```python
from build123d import *

# Parameters (mm, degrees)
BASE_EXTRUDE_DEPTH  = 2.54
SKETCH2_W           = 9.525
SKETCH2_H           = 6.35
CUT_EXTRUDE1_DEPTH  = 0.508
SKETCH3_W           = 4.572
SKETCH3_H           = 6.35
BOSS_EXTRUDE1_DEPTH = 8.382
SKETCH4_R           = 1.5875
CUT_EXTRUDE2_DEPTH  = 19.230583479
SKETCH5_W           = 4.1402
SKETCH5_H           = 5.08
BOSS_EXTRUDE2_DEPTH = 4.826
BOSS_EXTRUDE3_DEPTH = 0.635
SKETCH7_R           = 0.127
BOSS_EXTRUDE4_DEPTH = 9.525


with BuildPart() as part:
    # Sketch1 → Base-Extrude (new body)
    with BuildSketch(Plane(origin=(0, 0, 0), x_dir=(1, 0, 0), z_dir=(0, 1, 0))):
        with BuildLine():
            Line((12.7, 3.175), (-12.7, 3.175))
            ThreePointArc((-12.7, 3.175), (-15.875, 0), (-12.7, -3.175))
            Line((-12.7, -3.175), (12.7, -3.175))
            ThreePointArc((12.7, -3.175), (15.875, 0), (12.7, 3.175))
        make_face()
    extrude(amount=BASE_EXTRUDE_DEPTH)

    # Sketch2 → Cut-Extrude1 (cut)
    with BuildSketch(Plane(origin=(0, 2.54, 0), x_dir=(-1, 0, 0), z_dir=(0, 1, 0))):
        Rectangle(SKETCH2_W, SKETCH2_H)
    extrude(amount=-CUT_EXTRUDE1_DEPTH, mode=Mode.SUBTRACT)

    # Sketch3 → Boss-Extrude1 (add)
    with BuildSketch(Plane(origin=(0, 2.54, 0), x_dir=(-1, 0, 0), z_dir=(0, 1, 0))):
        with Locations((-7.0485, 0)):
            Rectangle(SKETCH3_W, SKETCH3_H)
        with Locations((7.0485, 0)):
            Rectangle(SKETCH3_W, SKETCH3_H)
    extrude(amount=BOSS_EXTRUDE1_DEPTH)

    # Sketch4 → Cut-Extrude2 (cut, through all)
    with BuildSketch(Plane(origin=(0, 2.54, 0), x_dir=(-1, 0, 0), z_dir=(0, 1, 0))):
        with Locations(Location((-12.7, 0, 0), (0, 0, 90))):
            Circle(SKETCH4_R)
        with Locations(Location((12.7, 0, 0), (0, 0, 270))):
            Circle(SKETCH4_R)
    extrude(amount=-CUT_EXTRUDE2_DEPTH, mode=Mode.SUBTRACT)

    # Sketch5 → Boss-Extrude2 (add)
    with BuildSketch(Plane.XZ):
        with Locations((6.1341, 0)):
            Rectangle(SKETCH5_W, SKETCH5_H)
        with Locations((-6.1341, 0)):
            Rectangle(SKETCH5_W, SKETCH5_H)
    extrude(amount=BOSS_EXTRUDE2_DEPTH)

    # Sketch6 → Boss-Extrude3 (add, symmetric)
    with BuildSketch(Plane.XY):
        with BuildLine():
            Line((-4.064, 0), (4.064, 0))
            Line((4.064, 0), (4.064, -3.305361967))
            ThreePointArc((4.064, -3.305361967), (0, -1.082087461), (-4.064, -3.305361967))
            Line((-4.064, -3.305361967), (-4.064, 0))
        make_face()
    extrude(amount=BOSS_EXTRUDE3_DEPTH, both=True)

    # Sketch7 → Boss-Extrude4 (add)
    with BuildSketch(Plane.ZY.offset(-4.7625)):
        with Locations(Location((0, 8.128, 0), (0, 0, 180))):
            Circle(SKETCH7_R)
    extrude(amount=BOSS_EXTRUDE4_DEPTH)


solid = part.part
```
Geometry: final body of the model. Coordinates: model frame, mm. A direction names the side the tool comes from. Round coordinates to 2 decimals unless told otherwise and drop trailing zeros. Write each loop counter-clockwise with the first axis right and the second up, starting at its lowest first coordinate (ties: lowest second). Pieces come first, ordered by that corner, then holes.
Item 1: Pin query (flat end, axial travel): P1, Ø1.2, axis at x = -6.5, y = -3, coming from the -Z side; P2, Ø2.5, axis at y = -2, z = -1, coming from the -X side; P3, Ø1, axis at x = 10.5, z = -0.5, coming from the -Y side. Return the tip coordinate at first contact, or that it passes through.
Item 2: Mould query, pull axis X, two halves, no side actions, for faces 1 (the face through (4.064, -3.5, 0)), 2 (the face through (-7, 10.922, 0)), 3 (the face through (-9.334, 7, 0)). Classes: +X half, -X half, draft (parallel to the pull), parting line (faces both ways), or undercut.
Item 3: Set-up query: faces 4 (the face through (6, -2, -2.54)), 5 (the face through (6, -2, 2.54)), 6 (the face through (-11, 2.54, 1)), 7 (the face through (9.334, 7, 0)), 8 (the face through (0.1, -0.9, 0.635)). Return all of +Z, -Z, +X, -X, +Y, -Y with unobstructed straight access to the full face (end or side cutting, diameter ignored); none if empty.
Item 4: Material intervals for L1, parallel to X at y = 1.45, z = 0 (1 decimal); L2, parallel to Z at x = -12.7, y = 1.1 (1 decimal); L3, parallel to X at y = -3.25, z = 2, sorted ascending.
Item 5: Section query B-B (z = -1). Return loops of the section in (x, y), plus the area to 3 significant figures.
Item 6: Section query D-D (y = -3). Return loops of the section in (x, z) (3 decimals).
Item 7: Section query C-C (x = -1). Return loops of the section in (y, z) (3 decimals).
Item 8: Section query A-A (y = 9.5). Return loops of the section in (x, z) (1 decimal), plus the area to 3 significant figures.
Completed:
1. P1: stops at z = -2.54
1. P2: stops at x = -8.2
1. P3: stops at y = 0
2. face 1: undercut
2. face 2: draft
2. face 3: -X half
3. face 4: -Z, +X, -X, -Y
3. face 5: +Z, +X, -X, -Y
3. face 6: +Z, -Z, -X, +Y
3. face 7: +Z, -Z, +X, +Y
3. face 8: +Z, -Y
4. L1: x = -15.9 to -14.3, -11.1 to 11.1, 14.3 to 15.9
4. L2: z = -3.2 to -1.6, 1.6 to 3.2
4. L3: x = -8.2 to -4.06, 4.06 to 8.2
5. outline: (-15.71, 0) - (-13.93, 0) - (-13.93, 2.54) - (-15.71, 2.54) - close; (-11.47, 0) - (-8.2, 0) - (-8.2, -4.83) - (-4.06, -4.83) - (-4.06, 0) - (4.06, 0) - (4.06, -4.83) - (8.2, -4.83) - (8.2, 0) - (11.47, 0) - (11.47, 2.54) - (9.33, 2.54) - (9.33, 10.92) - (4.76, 10.92) - (4.76, 2.03) - (-4.76, 2.03) - (-4.76, 10.92) - (-9.33, 10.92) - (-9.33, 2.54) - (-11.47, 2.54) - close; (13.93, 0) - (15.71, 0) - (15.71, 2.54) - (13.93, 2.54) - close
5. area: 179 mm2
6. outline: (-8.204, -2.54) - (-4.064, -2.54) - (-4.064, -0.635) - (-3.851, -0.635) - (-3.851, 0.635) - (-4.064, 0.635) - (-4.064, 2.54) - (-8.204, 2.54) - close; (3.851, -0.635) - (4.064, -0.635) - (4.064, -2.54) - (8.204, -2.54) - (8.204, 2.54) - (4.064, 2.54) - (4.064, 0.635) - (3.851, 0.635) - close
7. outline: (-1.187, -0.635) - (0, -0.635) - (0, -3.175) - (2.032, -3.175) - (2.032, 3.175) - (0, 3.175) - (0, 0.635) - (-1.187, 0.635) - close; circle Ø0.254 at (8.128, 0)
8. outline: (-9.3, -3.2) - (-4.8, -3.2) - (-4.8, 3.2) - (-9.3, 3.2) - close; (4.8, -3.2) - (9.3, -3.2) - (9.3, 3.2) - (4.8, 3.2) - close
8. area: 58.1 mm2
